```python
from build123d import *

# Parameters (mm, degrees)
BOX_W             = 69
BOX_H             = 23
BOX_DEPTH         = 21
FILLET002039_R    = 7
BOX048_W          = 69
BOX048_H          = 23
BOX048_DEPTH      = 21
CYLINDER_R        = 0.7
CYLINDER_DEPTH    = 25
CYLINDER042_R     = 0.7
CYLINDER042_DEPTH = 25
CYLINDER043_R     = 0.7
CYLINDER043_DEPTH = 25
CYLINDER044_R     = 0.7
CYLINDER044_DEPTH = 25
CYLINDER045_R     = 0.7
CYLINDER045_DEPTH = 25
CYLINDER046_R     = 0.7
CYLINDER046_DEPTH = 25
CYLINDER047_R     = 0.7
CYLINDER047_DEPTH = 25
CYLINDER048_R     = 0.7
CYLINDER048_DEPTH = 25
BOX044_W          = 83
BOX044_H          = 7
BOX044_DEPTH      = 10
FILLET002036_R    = 3
BOX029_W          = 83
BOX029_H          = 7
BOX029_DEPTH      = 18
FILLET002035_R    = 3
BOX045_W          = 10
BOX045_H          = 7
BOX045_DEPTH      = 14
BOX046_W          = 89
BOX046_H          = 23
BOX046_DEPTH      = 16
FILLET_R          = 4
FILLET002040_R    = 4


with BuildPart() as fillet002039:
    # Box → Box (new body)
    with BuildSketch(Plane(origin=(-42, -10, 0), x_dir=(1, 0, 0), z_dir=(0, 0, 1))):
        with Locations((34.5, 11.5)):
            Rectangle(BOX_W, BOX_H)
    extrude(amount=BOX_DEPTH)

    # Fillet002039
    fillet002039_edges = [fillet002039.edges().sort_by_distance(p)[0] for p in [
        (-7.5, -10, 21),
        (-7.5, 13, 21),
    ]]
    fillet(fillet002039_edges, radius=FILLET002039_R)


with BuildPart() as cut011004:
    # Box048 → Box048 (new body)
    with BuildSketch(Plane(origin=(-42, -10, 14), x_dir=(1, 0, 0), z_dir=(0, 0, 1))):
        with Locations((34.5, 11.5)):
            Rectangle(BOX048_W, BOX048_H)
    extrude(amount=BOX048_DEPTH)

    # Cut011004: cut Fillet002039
    add(fillet002039.part, mode=Mode.SUBTRACT)


with BuildPart() as obj1:
    # Cylinder → Cylinder (new body)
    with BuildSketch(Plane(origin=(-30, -6, 0), x_dir=(1, 0, 0), z_dir=(0, 0, 1))):
        Circle(CYLINDER_R)
    extrude(amount=CYLINDER_DEPTH)


with BuildPart() as obj2:
    # Cylinder042 → Cylinder042 (new body)
    with BuildSketch(Plane(origin=(-30, 9, 0), x_dir=(1, 0, 0), z_dir=(0, 0, 1))):
        Circle(CYLINDER042_R)
    extrude(amount=CYLINDER042_DEPTH)


with BuildPart() as obj3:
    # Cylinder043 → Cylinder043 (new body)
    with BuildSketch(Plane(origin=(15, -6, 0), x_dir=(1, 0, 0), z_dir=(0, 0, 1))):
        Circle(CYLINDER043_R)
    extrude(amount=CYLINDER043_DEPTH)


with BuildPart() as obj4:
    # Cylinder044 → Cylinder044 (new body)
    with BuildSketch(Plane(origin=(15, 9, 0), x_dir=(1, 0, 0), z_dir=(0, 0, 1))):
        Circle(CYLINDER044_R)
    extrude(amount=CYLINDER044_DEPTH)


with BuildPart() as obj5:
    # Cylinder045 → Cylinder045 (new body)
    with BuildSketch(Plane(origin=(-47, -6, 0), x_dir=(1, 0, 0), z_dir=(0, 0, 1))):
        Circle(CYLINDER045_R)
    extrude(amount=CYLINDER045_DEPTH)


with BuildPart() as obj6:
    # Cylinder046 → Cylinder046 (new body)
    with BuildSketch(Plane(origin=(-47, 9, 0), x_dir=(1, 0, 0), z_dir=(0, 0, 1))):
        Circle(CYLINDER046_R)
    extrude(amount=CYLINDER046_DEPTH)


with BuildPart() as obj7:
    # Cylinder047 → Cylinder047 (new body)
    with BuildSketch(Plane(origin=(32, 9, 0), x_dir=(1, 0, 0), z_dir=(0, 0, 1))):
        Circle(CYLINDER047_R)
    extrude(amount=CYLINDER047_DEPTH)


with BuildPart() as fusion033:
    # Cylinder048 → Cylinder048 (new body)
    with BuildSketch(Plane(origin=(32, -6, 0), x_dir=(1, 0, 0), z_dir=(0, 0, 1))):
        Circle(CYLINDER048_R)
    extrude(amount=CYLINDER048_DEPTH)

    # Fusion033: union obj1, obj2, obj3, obj4, obj5, obj6, obj7
    add(obj1.part)
    add(obj2.part)
    add(obj3.part)
    add(obj4.part)
    add(obj5.part)
    add(obj6.part)
    add(obj7.part)


with BuildPart() as fillet002036:
    # Box044 → Box044 (new body)
    with BuildSketch(Plane(origin=(-50, 0, 4), x_dir=(1, 0, 0), z_dir=(0, 0, 1))):
        with Locations((41.5, 3.5)):
            Rectangle(BOX044_W, BOX044_H)
    extrude(amount=BOX044_DEPTH)

    # Fillet002036
    fillet002036_edges = [fillet002036.edges().sort_by_distance(p)[0] for p in [
        (-8.5, 0, 4),
        (-8.5, 0, 14),
        (-8.5, 7, 4),
        (-8.5, 7, 14),
    ]]
    fillet(fillet002036_edges, radius=FILLET002036_R)


with BuildPart() as fillet002035:
    # Box029 → Box029 (new body)
    with BuildSketch(Plane.XY):
        with Locations((41.5, 3.5)):
            Rectangle(BOX029_W, BOX029_H)
    extrude(amount=BOX029_DEPTH)

    # Fillet002035
    fillet002035_edges = [fillet002035.edges().sort_by_distance(p)[0] for p in [
        (41.5, 0, 0),
        (41.5, 0, 18),
        (41.5, 7, 0),
        (41.5, 7, 18),
    ]]
    fillet(fillet002035_edges, radius=FILLET002035_R)


with BuildPart() as fusion034:
    # Box045 → Box045 (new body)
    with BuildSketch(Plane(origin=(83, 0, 2), x_dir=(1, 0, 0), z_dir=(0, 0, 1))):
        with Locations((5, 3.5)):
            Rectangle(BOX045_W, BOX045_H)
    extrude(amount=BOX045_DEPTH)

    # Fusion032: union Fillet002036, Fillet002035
    add(fillet002036.part)
    add(fillet002035.part)


with BuildPart() as fusion034_1:
    # Fusion032 placement: moved
    add(fusion034.part.moved(Location((-48, -2, 10))))

    # Fusion034: union Fusion033
    add(fusion033.part)


with BuildPart() as hubholder:
    # Box046 → Box046 (new body)
    with BuildSketch(Plane(origin=(-52, -10, 5), x_dir=(1, 0, 0), z_dir=(0, 0, 1))):
        with Locations((44.5, 11.5)):
            Rectangle(BOX046_W, BOX046_H)
    extrude(amount=BOX046_DEPTH)

    # Fillet
    fillet_edges = [hubholder.edges().sort_by_distance(p)[0] for p in [
        (-52, -10, 13),
        (-52, 13, 13),
        (37, -10, 13),
        (37, 13, 13),
    ]]
    fillet(fillet_edges, radius=FILLET_R)

    # Cut009: cut Fusion034
    add(fusion034_1.part, mode=Mode.SUBTRACT)

    # Cut011005: cut Cut011004
    add(cut011004.part, mode=Mode.SUBTRACT)

    # Fillet002040
    fillet002040_edges = [hubholder.edges().sort_by_distance(p)[0] for p in [
        (-42, -10, 17.5),
        (27, -10, 17.5),
        (27, 13, 17.5),
        (-42, 13, 17.5),
    ]]
    fillet(fillet002040_edges, radius=FILLET002040_R)


solid = hubholder.part
```
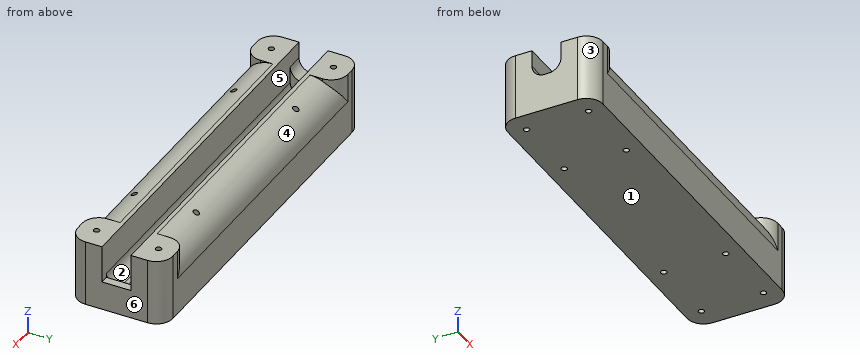
Build history of the part. All positions in model axes, mm. Face numbers are marked on the shaded views. A direction names the side the tool comes from. Round coordinates to 2 decimals unless told otherwise and drop trailing zeros. Loops run counter-clockwise (first coordinate to the right, second up) from the corner with the lowest first, then second, coordinate; pieces in that order, holes last.
Item 1: Saw through at B-B (y = 11). List the corners of the cut face in (x, z), then the cut area to 3 significant figures.
Item 2: Which spindle directions (+Z, -Z, +X, -X, +Y, -Y) get a long thin tool onto all of the face, cutting with end or side? Do the marked faces 1 and 2. Say none if no direction does.
Item 3: Saw through at A-A (z = 18.75). State how many separate pieces and enclosed holes the cut face has, then the cut area to 3 significant figures.
Item 4: Saw through at C-C (x = -45). List the corners of the cut face in (y, z), then the cut area to 3 significant figures.
Item 5: Pin check, flat tips, straight feed: P1, Ø1.1, axis at x = -30, y = -6, coming from the +Z side; P2, Ø1.6, axis at x = -30, y = 9, coming from the +Z side; P3, Ø5, axis at x = -1, z = 19, coming from the +Y side. Stop position of each tip, or through.
Item 6: Two-plate mould, pull along Y, no slides. Class the marked faces 3, 4, 5 and 6: released by +Y, released by -Y, zero draft, split by the parting line, or undercut.
Item 7: Drill centre lines: line 1 along Y through (x, z) = (-47, 13.75); line 2 along X through (y, z) = (9, 10.5); line 3 along Y through (x, z) = (15, 8). Where is each one in solid material? Low to high.
Worked answers:
1. outline: (-51.46, 5) - (36.46, 5) - (36.46, 21) - (27.54, 21) - (27.54, 18.9) - (-42.54, 18.9) - (-42.54, 21) - (-51.46, 21) - close
1. area: 1,260 mm2
2. face 1: -Z, +X, -X, +Y, -Y
2. face 2: +Z
3. separate pieces: 2
3. enclosed holes: 8
3. area: 1,130 mm2
4. outline: (-10, 5) - (13, 5) - (13, 14) arc R7 ccw to (12.87, 15.33) - (12.87, 21) - (5, 21) - (5, 13) arc R3 cw to (2, 10) - (1, 10) arc R3 cw to (-2, 13) - (-2, 21) - (-9.87, 21) - (-9.87, 15.33) arc R7 ccw to (-10, 14) - close
4. area: 293 mm2
5. P1: passes through
5. P2: stops at z = 20.65
5. P3: stops at y = 12.54
6. face 3: released by -Y
6. face 4: released by +Y
6. face 5: undercut
6. face 6: zero draft
7. line 1: y = -10 to -6.7, -5.3 to -2, 5 to 8.3, 9.7 to 13
7. line 2: x = -52 to -47.7, -46.3 to -30.7, -29.3 to 14.3, 15.7 to 31.3, 32.7 to 37
7. line 3: y = -10 to -6.7, -5.3 to 8.3, 9.7 to 13
